Part model, mm, in its own coordinate system. Give positions to 0.01 mm unless a question says otherwise; leave off trailing zeros. Write each loop counter-clockwise with the first axis right and the second up, starting at its lowest first coordinate (ties: lowest second). Pieces come first, ordered by that corner, then holes. Notation, with made-up numbers: M 88,60.5 L 105,60.5 A13 ccw 105,77.5 Z; hole C -25.5,88.5 d3. An arc over 180 degrees is marked long. Answer as CSV lines item,"result". Start each with the question number.
Item 1: Band-saw the part on B-B, the plane y = -73. List the corners of the cut face in (x, z).
Item 2: Band-saw the part on A-A, the plane z = -3. List the corners of the cut face in (x, y), then the cut area to 3 significant figures.
Item 3: Pin check, flat tips, straight feed: pin 1 (1.5 mm diameter, centred on y = -65, z = -1.5, fed in from +X); pin 2 (1 mm diameter, centred on y = -116, z = -2, fed in from +X); pin 3 (1 mm diameter, centred on y = -92, z = -1.5, fed in from +X). Stop position of each tip, or through.
Item 4: Band-saw the part on C-C, the plane x = 69.5. List the corners of the cut face in (y, z).
Item 5: Wall check: L1, parallel to Y at x = 75.5, z = -0.5; L2, parallel to Y at x = 86.5, z = -0.5; L3, parallel to X at y = -59, z = -0.75. Give the ranges that are in metal, low to high. Write a range as from..to.
Autodesk Inventor part; units mm, degrees
ref_plane "YZ Plane" through (0, 0, 0) normal (1, 0, 0) x (0, 1, 0)
ref_plane "XZ Plane" through (0, 0, 0) normal (0, 1, 0) x (-1, 0, 0)
ref_plane "XY Plane" through (0, 0, 0) normal (0, 0, 1) x (1, 0, 0)
sketch "Sketch1" plane through (0, 0, 0) normal (0, 0, 1) x (1, 0, 0)
  line L0 (0, 0) -> (0, -152.4)
  line L1 (0, -152.4) -> (38.1, -152.4)
  arc A0 (152.4, -38.1) -> (38.1, -152.4) centre (152.4, -152.4) ccw
  line L2 (152.4, -38.1) -> (152.4, 0)
  line L3 (152.4, 0) -> (0, 0)
  dimension "d0" = 152.4
  dimension "d1" = 152.4
  dimension "d2" = 38.1
  dimension "d3" = 38.1
extrude "Extrusion1" add sketch "Sketch1" against normal blind 6.35
properties part number "support"
Output:
1,outline,"M 0,-6.35 L 70.18,-6.35 L 70.18,0 L 0,0 Z"
2,outline,"M 0,-152.4 L 38.1,-152.4 A114.3 cw 152.4,-38.1 L 152.4,0 L 0,0 Z"
2,area,"13,000 mm²"
3,pin 1,"x = 79.64"
3,pin 2,"x = 44.22"
3,pin 3,"x = 55.68"
4,outline,"M -73.71,-6.35 L 0,-6.35 L 0,0 L -73.71,0 Z"
5,L1,"-67.84..0"
5,L2,"-59.01..0"
5,L3,"0..86.51"
